Part model, mm, in its own coordinate system. A direction names the side the tool comes from. Round coordinates to 2 decimals unless told otherwise and drop trailing zeros. Order: outer loops, then holes, each group sorted by start corner. A loop starts at its lowest first (then second) coordinate and runs counter-clockwise, first axis right, second up. Notation, with made-up numbers: (70, 5) - (125, 5) arc R33 cw to (125, 36) - close; hole circle Ø8 at (-37, 78.25). An arc over 180 degrees is marked (long way). Return JSON: item names as keys, results as strings. Group by question number.
Item 1: Probe probe 1 along Z at (x, y) = (5.5, 63); probe 2 along Z at (x, y) = (3, 12); probe 3 along Z at (x, y) = (2.5, 41.5). List the from-to ranges inside material, lowest first.
Item 2: Tool access for faces 1 (the face through (1, 74, -2)), 2 (the face through (3.313, 36, -5)), 3 (the face through (2.263, 36, -3)): list every direction of +Z, -Z, +X, -X, +Y, -Y with a clear straight run to the whole face (end or side of a thin tool).
Item 3: Drop flat-ended pins along their axis: pin 1 (5 mm diameter, centred on x = 10, y = 40, fed in from -Z); pin 2 (0.7 mm diameter, centred on y = 38, z = -3.5, fed in from -X); pin 3 (1 mm diameter, centred on x = -5, y = 37.5, fed in from -Z). Give the stop position or say it passes through.
Item 4: Two-plate mould, pull along Z, no slides. Class faces 4 (the face through (-2.187, 36, -5)), 5 (the face through (-1.137, 36, -3)), 6 (the face through (1, 36, -6.518)): released by +Z, released by -Z, zero draft, split by the parting line, or undercut.
Item 5: Saw through at A-A on y = 34.5. List the corners of the cut face in (x, z), and give its area (3 significant figures).
Item 6: Saw through at B-B on z = -5.5. List the corners of the cut face in (x, y).
```python
from build123d import *

# Parameters (mm, degrees)
BOSS_EXTRUDE1_DEPTH = 74
FILLET2_R           = 1
FILLET3_R           = 0.2


with BuildPart() as part:
    # Sketch4 → Boss-Extrude1 (new body)
    with BuildSketch(Plane(origin=(0, 0, 0), x_dir=(1, 0, 0), z_dir=(0, 1, 0))):
        Polygon((2.263347742, 4.418167116), (2.263347742, 1.178167116), (13.063347742, 0.388167116), (13.063347742, -0.321832884), (-11.936652258, -0.321832884), (-11.936652258, 0.388167116), (-1.136652258, 1.178167116), (-1.136652258, 4.418167116), (-2.186652258, 4.418167116), (-2.186652258, 6.518167116), (3.313347742, 6.518167116), (3.313347742, 4.418167116), align=None)
    extrude(amount=BOSS_EXTRUDE1_DEPTH)

    # Fillet2
    fillet2_edges = [part.edges().sort_by_distance(p)[0] for p in [
        (-1.136652258, 37, -1.178167116),
        (2.263347742, 37, -1.178167116),
    ]]
    fillet(fillet2_edges, radius=FILLET2_R)

    # Fillet3
    fillet3_edges = [part.edges().sort_by_distance(p)[0] for p in [
        (0.563347742, 74, -6.518167116),
        (-1.136652258, 0, -3.26292892),
        (-7.000175641, 0, -0.749261239),
        (-11.936652258, 0, -0.033167116),
        (0.563347742, 0, 0.321832884),
        (13.063347742, 0, -0.033167116),
        (3.313347742, 74, -5.468167116),
        (2.263347742, 0, -3.26292892),
        (2.788347742, 0, -4.418167116),
        (3.313347742, 0, -5.468167116),
        (0.563347742, 0, -6.518167116),
        (-2.186652258, 0, -5.468167116),
        (-1.661652258, 0, -4.418167116),
        (2.788347742, 74, -4.418167116),
        (2.263347742, 74, -3.26292892),
        (3.313347742, 37, -4.418167116),
        (3.313347742, 37, -6.518167116),
        (-2.186652258, 37, -6.518167116),
        (-2.186652258, 37, -4.418167116),
        (13.063347742, 74, -0.033167116),
        (0.563347742, 74, 0.321832884),
        (-11.936652258, 74, -0.033167116),
        (-7.000175641, 74, -0.749261239),
        (8.126871124, 0, -0.749261239),
        (8.126871124, 74, -0.749261239),
        (-1.136652258, 74, -3.26292892),
        (2.5309021, 0, -1.426865209),
        (2.5309021, 74, -1.426865209),
        (-1.404206617, 0, -1.426865209),
        (-1.404206617, 74, -1.426865209),
        (-1.661652258, 74, -4.418167116),
        (-2.186652258, 74, -5.468167116),
    ]]
    fillet(fillet3_edges, radius=FILLET3_R)


solid = part.part
```
Filled in:
{
 "1": {"probe 1": "z = -0.94 to 0.32", "probe 2": "z = -6.52 to -4.42, -1.14 to 0.32", "probe 3": "z = -6.52 to -4.42, -1.46 to 0.32"},
 "2": {"face 1": "+Z, -Z, +X, -X, +Y", "face 2": "-Z, +X, +Y, -Y", "face 3": "+X, +Y, -Y"},
 "3": {"pin 1": "stops at z = -0.8", "pin 2": "stops at x = -1.14", "pin 3": "stops at z = -0.93"},
 "4": {"face 4": "zero draft", "face 5": "undercut", "face 6": "released by -Z"},
 "5": {"outline": "(-11.94, -0.39) - (-2.06, -1.11) arc R1 cw to (-1.14, -2.11) - (-1.14, -4.42) - (-1.99, -4.42) arc R0.2 ccw to (-2.19, -4.62) - (-2.19, -6.32) arc R0.2 ccw to (-1.99, -6.52) - (3.11, -6.52) arc R0.2 ccw to (3.31, -6.32) - (3.31, -4.62) arc R0.2 ccw to (3.11, -4.42) - (2.26, -4.42) - (2.26, -2.11) arc R1 cw to (3.19, -1.11) - (13.06, -0.39) - (13.06, 0.32) - (-11.94, 0.32) - close", "area": "51.9 mm^2"},
 "6": {"outline": "(-2.19, 0.2) arc R0.2 ccw to (-1.99, 0) - (3.11, 0) arc R0.2 ccw to (3.31, 0.2) - (3.31, 73.8) arc R0.2 ccw to (3.11, 74) - (-1.99, 74) arc R0.2 ccw to (-2.19, 73.8) - close"}
}
